Solid Edge part; units mm, degrees
sketch "Sketch1" plane through (0, 0, 0) normal (0, 0, 1) x (1, 0, 0)
  line L0 (14.3615, 4.5) -> (19.1615, 4.5)
  arc A0 (19.1615, 4.5) -> (22.6615, 1) centre (19.1615, 1) cw
  line L1 (22.6615, 1) -> (22.6615, -1)
  arc A1 (22.6615, -1) -> (19.1615, -4.5) centre (19.1615, -1) cw
  line L2 (19.1615, -4.5) -> (14.3615, -4.5)
  arc A2 (14.3615, -4.5) -> (14.121, -5.2058) centre (0, 0) cw
  line L3 (14.121, -5.2058) -> (13.05, -5.2058)
  arc A3 (0, 14.05) -> (-13.05, -5.2058) centre (0, 0) ccw
  line L4 (-14.121, -5.2058) -> (-13.05, -5.2058)
  arc A4 (-14.3615, -4.5) -> (-14.121, -5.2058) centre (0, 0) ccw
  line L5 (-19.1615, -4.5) -> (-14.3615, -4.5)
  arc A5 (-22.6615, -1) -> (-19.1615, -4.5) centre (-19.1615, -1) ccw
  line L6 (-22.6615, 1) -> (-22.6615, -1)
  arc A6 (-19.1615, 4.5) -> (-22.6615, 1) centre (-19.1615, 1) ccw
  line L7 (-14.3615, 4.5) -> (-19.1615, 4.5)
  arc A7 (0, 15.05) -> (-14.3615, 4.5) centre (0, 0) ccw
  arc A8 (0, 15.05) -> (14.3615, 4.5) centre (0, 0) cw
  arc A9 (0, 14.05) -> (13.05, -5.2058) centre (0, 0) cw
extrude "Protrusion1" add sketch "Sketch1" along normal blind 10
sketch "Sketch2" plane through (0, 4.9221, 10) normal (0, 0, 1) x (1, 0, 0)
  circle A0 centre (17.5015, -4.9221) radius 2.1
  circle A1 centre (-17.5015, -4.9221) radius 2.1
extrude "Wycięcie_3" cut sketch "Sketch2" against normal blind 2.4
fillet "Zaokrąglenie_2" [suppressed]
sketch "Sketch3" plane through (0, 4.9221, 0) normal (0, 0, -1) x (-1, 0, 0)
  arc A0 (6.55, 10.1279) -> (8.91, 7.2069) centre (13.2727, 13.1457) ccw
  arc A1 (0, 10.1279) -> (8.91, 7.2069) centre (0, -4.9221) cw
  arc A2 (0, 10.1279) -> (-8.91, 7.2069) centre (0, -4.9221) ccw
  arc A3 (-6.55, 10.1279) -> (-8.91, 7.2069) centre (-13.2727, 13.1457) cw
  line L0 (-6.55, 10.1279) -> (-6.55, 15.6279)
  line L1 (-6.55, 15.6279) -> (-0.05, 15.6279)
  line L2 (-0.05, 14.1279) -> (-0.05, 15.6279)
  line L3 (-5.05, 14.1279) -> (-0.05, 14.1279)
  line L4 (-5.05, 11.1279) -> (-5.05, 14.1279)
  line L5 (0, 11.1279) -> (-5.05, 11.1279)
  line L6 (0, 11.1279) -> (5.05, 11.1279)
  line L7 (5.05, 11.1279) -> (5.05, 14.1279)
  line L8 (5.05, 14.1279) -> (0.05, 14.1279)
  line L9 (0.05, 14.1279) -> (0.05, 15.6279)
  line L10 (6.55, 15.6279) -> (0.05, 15.6279)
  line L11 (6.55, 10.1279) -> (6.55, 15.6279)
extrude "Protrusion2" add sketch "Sketch3" against normal up to vertex (10 mm away)
sketch "Sketch4" plane through (0, 4.9221, 0) normal (0, 0, -1) x (-1, 0, 0)
  arc A0 (-14.3615, -0.4221) -> (-8.91, 7.2069) centre (0, -4.9221) cw
  arc A1 (-6.55, 10.1279) -> (-8.91, 7.2069) centre (-13.2727, 13.1457) cw
  line L0 (-6.55, 10.1279) -> (-6.55, 15.6279)
  line L1 (-6.55, 15.6279) -> (-0.05, 15.6279)
  line L2 (-0.05, 14.1279) -> (-0.05, 15.6279)
  line L3 (-5.05, 14.1279) -> (-0.05, 14.1279)
  line L4 (-5.05, 11.1279) -> (-5.05, 14.1279)
  line L5 (0, 11.1279) -> (-5.05, 11.1279)
  line L6 (0, 11.1279) -> (5.05, 11.1279)
  line L7 (5.05, 11.1279) -> (5.05, 14.1279)
  line L8 (5.05, 14.1279) -> (0.05, 14.1279)
  line L9 (0.05, 14.1279) -> (0.05, 15.6279)
  line L10 (6.55, 15.6279) -> (0.05, 15.6279)
  line L11 (6.55, 10.1279) -> (6.55, 15.6279)
  arc A2 (6.55, 10.1279) -> (8.91, 7.2069) centre (13.2727, 13.1457) ccw
  arc A3 (8.91, 7.2069) -> (14.3615, -0.4221) centre (0, -4.9221) cw
  line L12 (14.3615, -0.4221) -> (19.1615, -0.4221)
  arc A4 (19.1615, -0.4221) -> (22.6615, -3.9221) centre (19.1615, -3.9221) cw
  line L13 (22.6615, -3.9221) -> (22.6615, -5.9221)
  arc A5 (22.6615, -5.9221) -> (19.1615, -9.4221) centre (19.1615, -5.9221) cw
  line L14 (19.1615, -9.4221) -> (14.3615, -9.4221)
  arc A6 (14.3615, -9.4221) -> (14.121, -10.1279) centre (0, -4.9221) cw
  line L15 (14.121, -10.1279) -> (13.05, -10.1279)
  arc A7 (13.05, -10.1279) -> (-13.05, -10.1279) centre (0, -4.9221) ccw
  line L16 (-13.05, -10.1279) -> (-14.121, -10.1279)
  arc A8 (-14.121, -10.1279) -> (-14.3615, -9.4221) centre (0, -4.9221) cw
  line L17 (-14.3615, -9.4221) -> (-19.1615, -9.4221)
  arc A9 (-19.1615, -9.4221) -> (-22.6615, -5.9221) centre (-19.1615, -5.9221) cw
  line L18 (-22.6615, -5.9221) -> (-22.6615, -3.9221)
  arc A10 (-22.6615, -3.9221) -> (-19.1615, -0.4221) centre (-19.1615, -3.9221) cw
  line L19 (-19.1615, -0.4221) -> (-14.3615, -0.4221)
extrude "Wycięcie_8" add sketch "Sketch4" along normal blind 5
sketch "Sketch5" plane through (0, 7.6721, 8.5) normal (0, 0, 1) x (1, 0, 0)
  line L0 (-17.6, -4.1679) -> (-13.05, -4.1679)
  line L1 (-13.05, -4.1679) -> (-13.05, -11.5863)
  line L2 (-13.05, -11.5863) -> (-17.6, -11.5863)
  arc A0 (-17.6, -11.5863) -> (-21.1, -8.0863) centre (-17.6, -8.0863) cw
  line L3 (-21.1, -8.0863) -> (-21.1, -7.6679)
  arc A1 (-17.6, -4.1679) -> (-21.1, -7.6679) centre (-17.6, -7.6679) ccw
  arc A2 (17.6, -4.1679) -> (21.1, -7.6679) centre (17.6, -7.6679) cw
  line L4 (21.1, -8.0863) -> (21.1, -7.6679)
  arc A3 (17.6, -11.5863) -> (21.1, -8.0863) centre (17.6, -8.0863) ccw
  line L5 (13.05, -11.5863) -> (17.6, -11.5863)
  line L6 (13.05, -4.1679) -> (13.05, -11.5863)
  line L7 (17.6, -4.1679) -> (13.05, -4.1679)
extrude "Cutout1" cut sketch "Sketch5" against normal blind 1.2
chamfer "Faza_3" distance 0.4 angle 45 10 edges at (-15.603, 3.5042, 8.5) (-20.0749, 2.4791, 8.5) (-21.1, -0.205, 8.5) (-20.0749, -2.889, 8.5) (-15.5469, -3.9141, 8.5) (15.603, 3.5042, 8.5) (20.0749, 2.4791, 8.5) (21.1, -0.205, 8.5) (20.0749, -2.889, 8.5) (15.5469, -3.9141, 8.5)
sketch "Sketch6" plane through (-17.2969, -0.205, 7.3) normal (0, 0, 1) x (1, 0, 0)
  circle A0 centre (-0.2046, 0.205) radius 2.1
  circle A1 centre (34.7984, 0.205) radius 2.1
extrude "Wyciągnięcie_7" add sketch "Sketch6" along normal blind 0.3
chamfer "Faza_4" distance 0.3 angle 45 2 edges at (-19.6015, 0, 7.6) (15.4015, 0, 7.6)
sketch "Sketch7" plane through (-17.2969, -0.205, 7.3) normal (0, 0, 1) x (1, 0, 0)
  circle A0 centre (2.6056, 0.205) radius 0.15
  circle A1 centre (-2.9586, 0.205) radius 0.15
  circle A2 centre (31.9882, 0.205) radius 0.15
  circle A3 centre (37.5524, 0.205) radius 0.15
extrude "Protrusion3" add sketch "Sketch7" along normal up to vertex (1.2 mm away)
sketch "Sketch8" plane through (-17.5015, 0, 7.6) normal (0, 0, 1) x (1, 0, 0)
  circle A0 centre (0, 0) radius 1.5
  circle A1 centre (35.003, 0) radius 1.5
extrude "Cutout2" cut sketch "Sketch8" against normal through all
For this review, take the finished solid that the model builds, in its own axes (mm). A direction names the side the tool comes from. Give positions to 0.01 mm unless a question says otherwise; leave off trailing zeros. Write each loop counter-clockwise with the first axis right and the second up, starting at its lowest first coordinate (ties: lowest second). Pieces come first, ordered by that corner, then holes. Notation, with made-up numbers: M 45.25,-0.75 L 77.25,-0.75 A26 cw 77.25,35.25 Z; hole C 23.25,72.5 d3. An arc over 180 degrees is marked long. One line per item, written item: value.
1) Take a section at C-C, the plane z = -2. Count the separate pieces of the cut face and the enclosed holes in it, then the cut area to 3 significant figures.
Results are:
separate pieces: 1
enclosed holes: 2
area: 223 mm²
2) For faces 1 (the flat face through (-17, 4.5, 2)), 2 (the conical face through (-19.897, 2.252, 8.386)), 3 (the flat face through (-3, 19.05, 2)), list the 3-axis set-ups (+Z, -Z, +X, -X, +Y, -Y) from which the entire face can be reached by the end or side of a thin tool; tool diameter is ignored.
Results are:
face 1: +Z, -Z, -X, +Y
face 2: none
face 3: +Z, -Z
3) The part is to be moulded in two halves that separate along Y. For faces 4 (the cylindrical face through (21.61, 3.5, 2.39)), 5 (the flat face through (-5.05, 18, 2)), 6 (the flat face through (13.6, -5.206, 2.4)), say which applies: +Y half, -Y half, draft (parallel to the pull), parting line (faces both ways), or undercut.
Results are:
face 4: +Y half
face 5: undercut
face 6: -Y half
4) Take a section at B-B, the plane y = 5.5. Write out the cut boundary in (x, z), then the cut area to 3 significant figures.
Results are:
outline: M -14.01,-5 L -12.93,-5 L -12.93,10 L -14.01,10 Z; M 12.93,-5 L 14.01,-5 L 14.01,10 L 12.93,10 Z
area: 32.4 mm²
5) For line 1 (Y direction, x = -3.5, z = -1.75); line 2 (X direction, y = 17.5, z = 1.25); line 3 (Y direction, x = 0, z = 5), list the stretches that pass through material, from the lowest coordinate up. Write a range as from..to.
Results are:
line 1: y = 13.61..16.05, 19.05..20.55
line 2: x = -6.55..-5.05, 5.05..6.55
line 3: y = 14.05..16.05
6) For P1, Ø2.5, axis at y = 17.5, z = 3.5, coming from the +X side; P2, Ø1.4, axis at x = -17.5, z = 3.5, coming from the -Y side; P3, Ø2.5, axis at x = 17.5, y = 0, coming from the -Z side; P4, Ø1.5, axis at y = 18, z = 2.5, coming from the -X side, all flat-tipped, find the tip position at first contact; note any pin that passes through.
Results are:
P1: stops at x = 6.55
P2: stops at y = -4.5
P3: passes through
P4: stops at x = -6.55
7) Take a section at A-A, the plane x = 1. Write out the cut boundary in (y, z).
Results are:
outline: M 14.01,-5 L 16.05,-5 L 16.05,10 L 14.01,10 Z; M 19.05,-5 L 20.55,-5 L 20.55,10 L 19.05,10 Z
